from build123d import *

# Parameters (mm, degrees)
F0_W     = 44.45
F0_H     = 12.7
F2_W     = 31.75
F2_H     = 25.4
F3_DEPTH = 88.901
F5_W     = 22.225
F5_H     = 38.1
F6_DEPTH = 125.0798323142


with BuildPart() as f1:
    # F0 (on Front) → F1 (revolve)
    with BuildSketch(Plane.XZ):
        with Locations((0, 82.55)):
            Rectangle(F0_W, F0_H)
    revolve(axis=Axis((0, 0, 0), (1, 0, 0)))

    # F2 (on Front) → F3 (cut, through all)
    with BuildSketch(Plane.XZ):
        with Locations((15.875, 0)):
            Rectangle(F2_W, F2_H)
        with Locations((-15.875, 0)):
            Rectangle(F2_W, F2_H)
    extrude(amount=F3_DEPTH, mode=Mode.SUBTRACT)

    # F5 (on face) → F6 (cut, through all)
    with BuildSketch(Plane(origin=(0, 0, 0), x_dir=(1, 0, 0), z_dir=(0, -0.7071067812, -0.7071067812))):
        with Locations((11.1125, 0)):
            Rectangle(F5_W, F5_H)
    extrude(amount=F6_DEPTH, mode=Mode.SUBTRACT)


solid = f1.part
Geometry: final body of the model. Coordinates: model frame, mm. A direction names the side the tool comes from. Round coordinates to 2 decimals unless told otherwise and drop trailing zeros. Loops run counter-clockwise (first coordinate to the right, second up) from the corner with the lowest first, then second, coordinate; pieces in that order, holes last.
Q1. Pull-direction query (Y, two-part tool) for faces 1 (the cylindrical face through (0.31, 88.82, -3.73)), 2 (the flat face through (10.96, -43.25, -70.19)), 3 (the cylindrical face through (0.311, 76.134, -3.172)); classes: released by +Y, released by -Y, zero draft, split by the parting line, or undercut.
Q2. Section B-B on x = 4. Return loops of the section in (y, z).
Q3. Section A-A on y = 0. Return loops of the section in (x, z) (3 decimals), plus the area to 3 significant figures.
Q4. Access query for faces 4 (the flat face through (10.96, -70.19, -43.25)), 5 (the flat face through (0, -57, -58)), 6 (the flat face through (-22.225, 72, 27)), 7 (the flat face through (0, -81, 12.7)), 8 (the flat face through (22.225, -77, -30)). Directions: +Z, -Z, +X, -X, +Y, -Y. A direction counts if a zero-diameter tool reaches every point of the face in a straight line with its end or side. Return the directions, or none.
Q5. Section C-C on y = -43.5. Return loops of the section in (x, z) (3 decimals), plus the area to 3 significant figures.
Q6. Section D-D on z = 0. Return loops of the section in (x, y) (3 decimals).
Q7. Material intervals for L1, parallel to Z at x = 8, y = 0; L2, parallel to Y at x = 9, z = 0; L3, parallel to Z at x = -17, y = -41.5, sorted ascending.
Q8. Pin query (flat end, axial travel): P1, Ø6, axis at x = 13.5, z = 37, coming from the -Y side; P2, Ø4, axis at x = -17, z = -68, coming from the -Y side; P3, Ø4, axis at x = -8, y = -80.5, coming from the +Z side. Return the tip coordinate at first contact, or that it passes through.
Evaluation:
1. face 1: split by the parting line
1. face 2: released by -Y
1. face 3: undercut
2. outline: (-87.99, -12.7) arc R88.9 ccw to (-74.87, -47.93) - (-65.64, -38.7) arc R76.2 cw to (-75.13, -12.7) - close; (-87.99, 12.7) - (-75.13, 12.7) arc R76.2 cw (long way) to (-38.7, -65.64) - (-47.93, -74.87) arc R88.9 ccw (long way) to start
3. outline: (-22.225, -88.9) - (22.225, -88.9) - (22.225, -76.2) - (-22.225, -76.2) - close; (-22.225, 76.2) - (22.225, 76.2) - (22.225, 88.9) - (-22.225, 88.9) - close
3. area: 1,130 mm2
4. face 4: -Z, +X
4. face 5: +X
4. face 6: +Z, -Z, -X, +Y, -Y
4. face 7: +X, -X, -Y
4. face 8: +Z, -Z, +X, +Y, -Y
5. outline: (-22.225, -77.53) - (22.225, -77.53) - (22.225, -70.441) - (0, -70.441) - (0, -62.563) - (-22.225, -62.563) - close; (-22.225, 62.563) - (22.225, 62.563) - (22.225, 77.53) - (-22.225, 77.53) - close
5. area: 1,160 mm2
6. outline: (-22.225, 76.2) - (22.225, 76.2) - (22.225, 88.9) - (-22.225, 88.9) - close
7. L1: z = -88.9 to -76.2, 76.2 to 88.9
7. L2: y = 76.2 to 88.9
7. L3: z = -78.62 to -63.91, 63.91 to 78.62
8. P1: stops at y = -82.14
8. P2: stops at y = -59.56
8. P3: stops at z = 41.72
